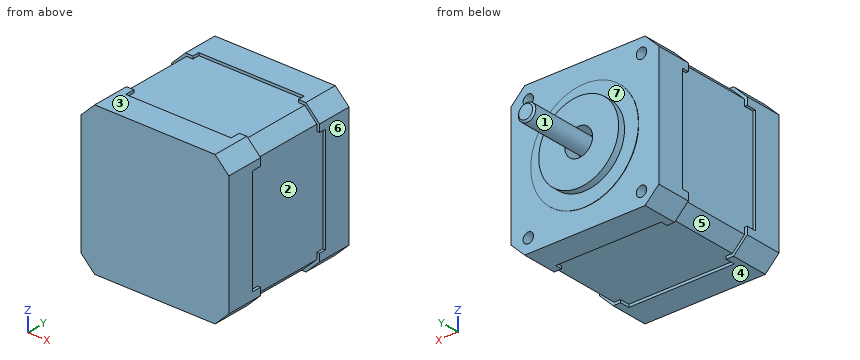
from build123d import *

# Parameters (mm, degrees)
SALIENTE_EXTRUIR2_DEPTH = 10
VACIADO6_T              = 0.78
CROQUIS2_W              = 30.346173158
CROQUIS2_H              = 2.78
CORTAR_EXTRUIR1_DEPTH   = 49.622957541
CROQUIS3_W              = 30.346173158
CROQUIS3_H              = 2.78
CORTAR_EXTRUIR2_DEPTH   = 49.622957541
SALIENTE_EXTRUIR3_DEPTH = 40
SALIENTE_EXTRUIR4_DEPTH = 10
CROQUIS6_W              = 30.346173158
CROQUIS6_H              = 2
CORTAR_EXTRUIR3_DEPTH   = 0.78
CROQUIS7_W              = 30.346173158
CROQUIS7_H              = 2
CORTAR_EXTRUIR4_DEPTH   = 0.78
CROQUIS8_W              = 30.346173158
CROQUIS8_H              = 2
CORTAR_EXTRUIR5_DEPTH   = 0.78
CROQUIS9_W              = 30.346173158
CROQUIS9_H              = 2
CORTAR_EXTRUIR6_DEPTH   = 0.78
CROQUIS10_R             = 1.5
CORTAR_EXTRUIR7_DEPTH   = 4
CROQUIS11_R             = 15.5
SALIENTE_EXTRUIR5_DEPTH = 0.1
CROQUIS12_R             = 11.5
SALIENTE_EXTRUIR6_DEPTH = 2
CROQUIS13_R             = 4
CORTAR_EXTRUIR8_DEPTH   = 5
CROQUIS14_R             = 2.5
SALIENTE_EXTRUIR7_DEPTH = 23
CHAFL_N1_SIZE           = 0.5


with BuildPart() as part:
    # Croquis1 → Saliente-Extruir2 (new body)
    with BuildSketch(Plane(origin=(0, 0, 0), x_dir=(1, 0, 0), z_dir=(0, 1, 0))):
        Polygon((20.5, 17), (17, 20.5), (-17, 20.5), (-20.5, 17), (-20.5, -17), (-17, -20.5), (17, -20.5), (20.5, -17), align=None)
    extrude(amount=SALIENTE_EXTRUIR2_DEPTH)

    # Vaciado6
    vaciado6_openings = [part.faces().sort_by_distance(p)[0] for p in [
        (0, 10, 0),
    ]]
    offset(amount=VACIADO6_T, openings=vaciado6_openings, kind=Kind.INTERSECTION)

    # Croquis2 → Cortar-Extruir1 (cut, through all)
    with BuildSketch(Plane(origin=(21.28, 0, 0), x_dir=(0, 0, -1), z_dir=(1, 0, 0))):
        with Locations((0, 8.61)):
            Rectangle(CROQUIS2_W, CROQUIS2_H)
    extrude(amount=-CORTAR_EXTRUIR1_DEPTH, mode=Mode.SUBTRACT)

    # Croquis3 → Cortar-Extruir2 (cut, through all)
    with BuildSketch(Plane.XY.offset(21.28)):
        with Locations((0, 8.61)):
            Rectangle(CROQUIS3_W, CROQUIS3_H)
    extrude(amount=-CORTAR_EXTRUIR2_DEPTH, mode=Mode.SUBTRACT)

    # Croquis4 → Saliente-Extruir3 (add)
    with BuildSketch(Plane(origin=(0, 0, 0), x_dir=(1, 0, 0), z_dir=(0, 1, 0))):
        Polygon((-17, 20.5), (17, 20.5), (20.5, 17), (20.5, -17), (17, -20.5), (-17, -20.5), (-20.5, -17), (-20.5, 17), align=None)
    extrude(amount=SALIENTE_EXTRUIR3_DEPTH)

    # Croquis5 → Saliente-Extruir4 (add)
    with BuildSketch(Plane(origin=(0, 40, 0), x_dir=(1, 0, 0), z_dir=(0, 1, 0))):
        Polygon((-21.28, 17.323086579), (-17.323086579, 21.28), (17.323086579, 21.28), (21.28, 17.323086579), (21.28, -17.323086579), (17.323086579, -21.28), (-17.323086579, -21.28), (-21.28, -17.323086579), align=None)
    extrude(amount=-SALIENTE_EXTRUIR4_DEPTH)

    # Croquis6 → Cortar-Extruir3 (cut)
    with BuildSketch(Plane.XY.offset(21.28)):
        with Locations((0, 31)):
            Rectangle(CROQUIS6_W, CROQUIS6_H)
    extrude(amount=-CORTAR_EXTRUIR3_DEPTH, mode=Mode.SUBTRACT)

    # Croquis7 → Cortar-Extruir4 (cut)
    with BuildSketch(Plane(origin=(0, 0, -21.28), x_dir=(-1, 0, 0), z_dir=(0, 0, -1))):
        with Locations((0, 31)):
            Rectangle(CROQUIS7_W, CROQUIS7_H)
    extrude(amount=-CORTAR_EXTRUIR4_DEPTH, mode=Mode.SUBTRACT)

    # Croquis8 → Cortar-Extruir5 (cut)
    with BuildSketch(Plane.ZY.offset(21.28)):
        with Locations((0, 31)):
            Rectangle(CROQUIS8_W, CROQUIS8_H)
    extrude(amount=-CORTAR_EXTRUIR5_DEPTH, mode=Mode.SUBTRACT)

    # Croquis9 → Cortar-Extruir6 (cut)
    with BuildSketch(Plane(origin=(21.28, 0, 0), x_dir=(0, 0, -1), z_dir=(1, 0, 0))):
        with Locations((0, 31)):
            Rectangle(CROQUIS9_W, CROQUIS9_H)
    extrude(amount=-CORTAR_EXTRUIR6_DEPTH, mode=Mode.SUBTRACT)

    # Croquis10 → Cortar-Extruir7 (cut)
    with BuildSketch(Plane(origin=(0, 40, 0), x_dir=(1, 0, 0), z_dir=(0, 1, 0))):
        with Locations(Location((-16.28, 17.323086579, 0), (0, 0, 270))):
            Circle(CROQUIS10_R)
        with Locations(Location((16.28, 17.323086579, 0), (0, 0, 270))):
            Circle(CROQUIS10_R)
        with Locations(Location((16.28, -17.323086579, 0), (0, 0, 270))):
            Circle(CROQUIS10_R)
        with Locations(Location((-16.28, -17.323086579, 0), (0, 0, 270))):
            Circle(CROQUIS10_R)
    extrude(amount=-CORTAR_EXTRUIR7_DEPTH, mode=Mode.SUBTRACT)

    # Croquis11 → Saliente-Extruir5 (add)
    with BuildSketch(Plane(origin=(0, 40, 0), x_dir=(1, 0, 0), z_dir=(0, 1, 0))):
        with Locations(Location((0, 0, 0), (0, 0, 90))):
            Circle(CROQUIS11_R)
    extrude(amount=SALIENTE_EXTRUIR5_DEPTH)

    # Croquis12 → Saliente-Extruir6 (add)
    with BuildSketch(Plane(origin=(0, 40.1, 0), x_dir=(1, 0, 0), z_dir=(0, 1, 0))):
        with Locations(Location((0, 0, 0), (0, 0, 270))):
            Circle(CROQUIS12_R)
    extrude(amount=SALIENTE_EXTRUIR6_DEPTH)

    # Croquis13 → Cortar-Extruir8 (cut)
    with BuildSketch(Plane(origin=(0, 42.1, 0), x_dir=(1, 0, 0), z_dir=(0, 1, 0))):
        with Locations(Location((0, 0, 0), (0, 0, 270))):
            Circle(CROQUIS13_R)
    extrude(amount=-CORTAR_EXTRUIR8_DEPTH, mode=Mode.SUBTRACT)

    # Croquis14 → Saliente-Extruir7 (add)
    with BuildSketch(Plane(origin=(0, 37.1, 0), x_dir=(1, 0, 0), z_dir=(0, 1, 0))):
        with Locations(Location((0, 0, 0), (0, 0, 270))):
            Circle(CROQUIS14_R)
    extrude(amount=SALIENTE_EXTRUIR7_DEPTH)

    # Chaflán1
    chafl_n1_edges = [part.edges().sort_by_distance(p)[0] for p in [
        (0, 60.1, -2.5),
    ]]
    chamfer(chafl_n1_edges, length=CHAFL_N1_SIZE)


solid = part.part
Input: part model. Units: mm. Frame: model coordinates. Face numbers are marked on the shaded views. A direction names the side the tool comes from. Coordinates: 2 decimals unless noted, no trailing zeros. Loops run counter-clockwise (first coordinate to the right, second up) from the corner with the lowest first, then second, coordinate; pieces in that order, holes last.
(1) First-contact query: pin 1 Ø1.5 at (x, z) = (-4.5, -3.5) entering from +Y; pin 2 Ø0.9 at (x, y) = (20.5, 8.5) entering from -Z; pin 3 Ø0.6 at (x, y) = (21, 31) entering from +Z; pin 4 Ø18.5 at (x, z) = (0, -4.5) entering from +Y. Flat tips, straight axial feed; report the tip coordinate or a pass-through.
(2) Section A-A on y = 31. Return the cut outline in (x, z).
(3) Section D-D on x = 5.5. Return the cut outline in (y, z).
(4) Set-up query: the marked faces 5, 6 and 7. Return all of +Z, -Z, +X, -X, +Y, -Y with unobstructed straight access to the full face (end or side cutting, diameter ignored); none if empty.
(5) Pull-direction query (Z, two-part tool) for the marked faces 1, 2, 3 and 4; classes: released by +Z, released by -Z, zero draft, split by the parting line, or undercut.
(6) Material intervals for probe 1 along X at (y, z) = (39, 0); probe 2 along X at (y, z) = (42, 0); probe 3 along Y at (x, z) = (16, 8), sorted ascending.
Data:
1. pin 1: stops at y = 42.1
1. pin 2: stops at z = -18.55
1. pin 3: stops at z = 17.9
1. pin 4: stops at y = 60.1
2. outline: (-21.28, -17.32) - (-17.32, -21.28) - (-15.17, -21.28) - (-15.17, -20.5) - (15.17, -20.5) - (15.17, -21.28) - (17.32, -21.28) - (21.28, -17.32) - (21.28, -15.17) - (20.5, -15.17) - (20.5, 15.17) - (21.28, 15.17) - (21.28, 17.32) - (17.32, 21.28) - (15.17, 21.28) - (15.17, 20.5) - (-15.17, 20.5) - (-15.17, 21.28) - (-17.32, 21.28) - (-21.28, 17.32) - (-21.28, 15.17) - (-20.5, 15.17) - (-20.5, -15.17) - (-21.28, -15.17) - close
3. outline: (-0.78, -21.28) - (7.22, -21.28) - (7.22, -20.5) - (32, -20.5) - (32, -21.28) - (40, -21.28) - (40, -14.49) - (40.1, -14.49) - (40.1, -10.1) - (42.1, -10.1) - (42.1, 10.1) - (40.1, 10.1) - (40.1, 14.49) - (40, 14.49) - (40, 21.28) - (32, 21.28) - (32, 20.5) - (7.22, 20.5) - (7.22, 21.28) - (-0.78, 21.28) - close
4. face 5: -Z, -X
4. face 6: +Z, -Z, +X, +Y, -Y
4. face 7: +Y
5. face 1: undercut
5. face 2: undercut
5. face 3: released by +Z
5. face 4: released by -Z
6. probe 1: x = -21.28 to -4, -2.5 to 2.5, 4 to 21.28
6. probe 2: x = -11.5 to -4, -2.5 to 2.5, 4 to 11.5
6. probe 3: y = -0.78 to 40
